Study the drawing (mm; zero at the part's minimum x, y, z) and answer. A direction names the side the tool comes from. Round coordinates to 2 decimals unless told otherwise and drop trailing zeros. Loops run counter-clockwise (first coordinate to the right, second up) from the corner with the lowest first, then second, coordinate; pieces in that order, holes last. Notation, with made-up numbers: (-11, 3) - (25, 3) arc R37 ccw to (25, 41) - close; hole circle Ø4 at (44, -36). An arc over 180 degrees is marked (long way). Use CSV: the item, a comma, the result in double quotes. Start each with the question number.
1. A tool of negligible diameter and unlimited length cuts with its end or side. For the marked faces 1, 2 and 3, from which of +Z, -Z, +X, -X, +Y, -Y can it reach the whole face along a straight path? Write none if from no direction.
2. Find section C-C (z = 53). Give the vertices of the cut face in (x, y) (3 decimals).
3. Find section B-B (x = 13.5). Give the vertices of the cut face in (y, z) (3 decimals).
4. Consider line 1 along Z through (x, y) = (23, 12) (3 decimals); line 2 along Y through (x, z) = (1.25, 31.5) (3 decimals); line 3 along Z through (x, y) = (7.5, 0.5). Determine where each line is inside the solid, lowest interval first.
5. Find section A-A (x = 7.25). Give the vertices of the cut face in (y, z) (1 decimal), and give its area (3 significant figures).
6. Given pin 1 Ø4 at (x, z) = (10, 20.5) entering from -Y; pin 2 Ø5 at (y, z) = (7.5, 42) entering from -X; pin 3 Ø1 at (y, z) = (2.5, 27) entering from -X; pin 4 Ø1 at (x, y) = (11.5, 0.5) entering from -Z, each flat-ended and moving along its own axis, determine where each tip first touches the part or whether it passes through.
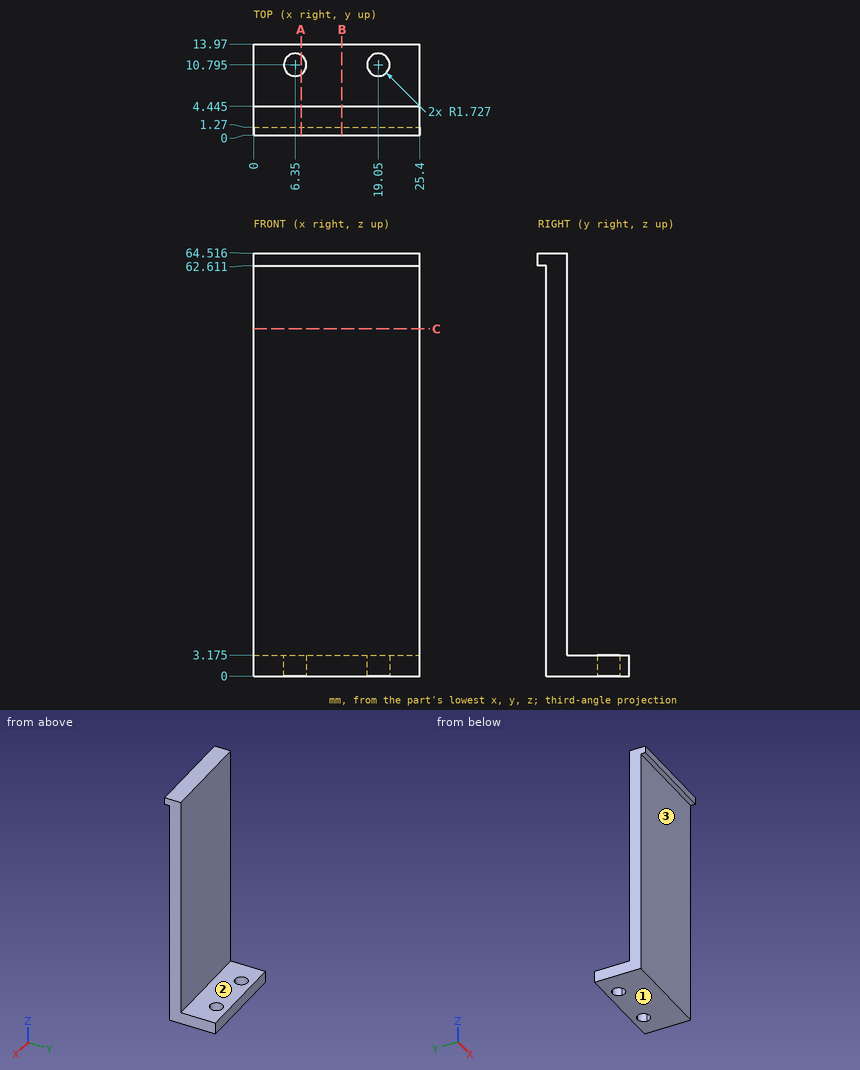
Filled sheet:
1,face 1,"-Z, +X, -X, +Y, -Y"
1,face 2,"+Z, +X, -X, +Y"
1,face 3,"-Z, +X, -X, -Y"
2,outline,"(0, 1.27) - (25.4, 1.27) - (25.4, 4.445) - (0, 4.445) - close"
3,outline,"(0, 62.611) - (1.27, 62.611) - (1.27, 0) - (13.97, 0) - (13.97, 3.175) - (4.445, 3.175) - (4.445, 64.516) - (0, 64.516) - close"
4,line 1,"z = 0 to 3.175"
4,line 2,"y = 1.27 to 4.445"
4,line 3,"z = 62.61 to 64.52"
5,outline,"(0, 62.6) - (1.3, 62.6) - (1.3, 0) - (9.3, 0) - (9.3, 3.2) - (4.4, 3.2) - (4.4, 64.5) - (0, 64.5) - close; (12.3, 0) - (14, 0) - (14, 3.2) - (12.3, 3.2) - close"
5,area,"228 mm²"
6,pin 1,"stops at y = 1.27"
6,pin 2,"passes through"
6,pin 3,"stops at x = 0"
6,pin 4,"stops at z = 62.61"
